from build123d import *

# Parameters (mm, degrees)
SKETCH3_W           = 49.53
SKETCH3_H           = 38.1
BOSS_EXTRUDE2_DEPTH = 7.62
SKETCH4_W           = 19.05
SKETCH4_H           = 12.7
CUT_EXTRUDE1_DEPTH  = 63.951531355
SKETCH6_R           = 1.651
CUT_EXTRUDE2_DEPTH  = 5.08
CUT_EXTRUDE3_START  = -5.08
SKETCH8_R           = 1.651
CUT_EXTRUDE3_DEPTH  = 5.08
FILLET3_R           = 7.62


with BuildPart() as part:
    # Sketch3 → Boss-Extrude2 (new body)
    with BuildSketch(Plane.XY):
        with Locations((24.765, 19.05)):
            Rectangle(SKETCH3_W, SKETCH3_H)
    extrude(amount=BOSS_EXTRUDE2_DEPTH)

    # Sketch4 → Cut-Extrude1 (cut, through all)
    with BuildSketch(Plane.XY.offset(7.62)):
        with Locations((26.035, 6.35)):
            Rectangle(SKETCH4_W, SKETCH4_H)
    extrude(amount=-CUT_EXTRUDE1_DEPTH, mode=Mode.SUBTRACT)

    # Sketch6 → Cut-Extrude2 (cut)
    with BuildSketch(Plane.XZ):
        with Locations(Location((8.255, 3.81, 0), (0, 0, 270))):
            Circle(SKETCH6_R)
        with Locations(Location((42.545, 3.81, 0), (0, 0, 270))):
            Circle(SKETCH6_R)
    extrude(amount=-CUT_EXTRUDE2_DEPTH, mode=Mode.SUBTRACT)

    # Sketch8 → Cut-Extrude3 (cut)
    with BuildSketch(Plane(origin=(0, 38.1, 0), x_dir=(1, 0, 0), z_dir=(0, 1, 0)).offset(CUT_EXTRUDE3_START)):
        with Locations(Location((8.255, -3.81, 0), (0, 0, 90))):
            Circle(SKETCH8_R)
        with Locations(Location((42.545, -3.81, 0), (0, 0, 90))):
            Circle(SKETCH8_R)
    extrude(amount=CUT_EXTRUDE3_DEPTH, mode=Mode.SUBTRACT)

    # Fillet3
    # the kernel refuses this fillet: 7.62 mm, written as the material it takes off along each edge
    with BuildSketch(Plane(origin=(49.53, -19.05, 7.62), x_dir=(-1, 0, 0), z_dir=(0, 1, 0))) as fillet3_piece_1:
        with BuildLine():
            CenterArc((FILLET3_R, -FILLET3_R), FILLET3_R, 90, 90)
            Line((0, -FILLET3_R), (0, 0))
            Line((0, 0), (FILLET3_R, 0))
        make_face()
    extrude(amount=76.2, mode=Mode.SUBTRACT)
    with BuildSketch(Plane(origin=(49.53, -19.05, 0), x_dir=(-1, 0, 0), z_dir=(0, 1, 0)), Plane(origin=(0, 57.15, 0), x_dir=(1, 0, 0), z_dir=(0, -1, 0)), Plane(origin=(0, 57.15, 7.62), x_dir=(0, 0, -1), z_dir=(0, -1, 0))) as fillet3_piece_2:
        with BuildLine():
            CenterArc((FILLET3_R, FILLET3_R), FILLET3_R, 180, 90)
            Line((0, FILLET3_R), (0, 0))
            Line((0, 0), (FILLET3_R, 0))
        make_face()
    extrude(amount=76.2, mode=Mode.SUBTRACT)


solid = part.part
Part model, mm, in its own coordinate system. A direction names the side the tool comes from. Coordinates: 2 decimals unless noted, no trailing zeros. Order: outer loops, then holes, each group sorted by start corner. A loop starts at its lowest first (then second) coordinate and runs counter-clockwise, first axis right, second up.
(1) Slice it at A-A, the plane y = 36.5. Write the cut outline in (x, z) (3 decimals).
Check sheet entries:
outline: (1.021, 3.81) arc R7.62 ccw to (7.62, 0) - (41.91, 0) arc R7.62 ccw to (48.509, 3.81) arc R7.62 ccw to (41.91, 7.62) - (7.62, 7.62) arc R7.62 ccw to start; hole circle Ø3.302 at (8.255, 3.81); hole circle Ø3.302 at (42.545, 3.81)
(2) Slice it at D-D, the plane x = 45. Write the cut outline in (y, z), and give its area (3 significant figures).
Check sheet entries:
outline: (0, 0.65) - (38.1, 0.65) - (38.1, 6.97) - (0, 6.97) - close
area: 240 mm2
(3) Slice it at B-B, the plane y = 22. Write the cut outline in (x, z), and give its area (3 significant figures).
Check sheet entries:
outline: (1.02, 3.81) arc R7.62 ccw to (7.62, 0) - (41.91, 0) arc R7.62 ccw to (48.51, 3.81) arc R7.62 ccw to (41.91, 7.62) - (7.62, 7.62) arc R7.62 ccw to start
area: 333 mm2
(4) Probe L1, parallel to X at y = 3.55, z = 3.81; L2, parallel to X at y = 36.85, z = 3.81; L3, parallel to X at y = 5, z = 3.25. List the from-to ranges inside material, lowest first.
Check sheet entries:
L1: x = 1.02 to 6.6, 9.91 to 16.51, 35.56 to 40.89, 44.2 to 48.51
L2: x = 1.02 to 6.6, 9.91 to 40.89, 44.2 to 48.51
L3: x = 1.38 to 6.7, 9.81 to 16.51, 35.56 to 40.99, 44.1 to 48.15
(5) Pin check, flat tips, straight feed: pin 1 Ø4 at (y, z) = (9, 5) entering from +X; pin 2 Ø2 at (x, z) = (42.545, 3.81) entering from -Y; pin 3 Ø1.7 at (x, z) = (8, 3.5) entering from +Y. Stop position of each tip, or through.
Check sheet entries:
pin 1: stops at x = 48.51
pin 2: stops at y = 5.08
pin 3: stops at y = 33.02
(6) Pull direction X, two halves, no side cores. Call faces 6 (the face through (25, 24, 0)), 7 (the face through (45.67, 18.78, 6.63)), 8 (the face through (44.182, 2.504, 4.025)): pulls with the +X half, pulls with the -X half, needs draft (parallel to the pull), parting line crosses it, or undercut.
Check sheet entries:
face 6: needs draft
face 7: pulls with the +X half
face 8: undercut
(7) Slice it at C-C, the plane z = 6.75. Write the cut outline in (x, y).
Check sheet entries:
outline: (4.08, 0) - (16.51, 0) - (16.51, 12.7) - (35.56, 12.7) - (35.56, 0) - (45.45, 0) - (45.45, 38.1) - (4.08, 38.1) - close
(8) Tool access for faces 1 (the face through (8, 5.08, 4)), 2 (the face through (44.157, 35.524, 4.168)), 3 (the face through (10.4, 0, 3.8)), 4 (the face through (24, 38.1, 4)), 5 (the face through (26, 12.7, 4)): list every direction of +Z, -Z, +X, -X, +Y, -Y with a clear straight run to the whole face (end or side of a thin tool).
Check sheet entries:
face 1: -Y
face 2: +Y
face 3: +Z, -Z, +X, -X, -Y
face 4: +Z, -Z, +X, -X, +Y
face 5: +Z, -Z, -Y
